from build123d import *

# Parameters (mm, degrees)
SKETCH1_W                            = 76.2
SKETCH1_H                            = 63.5
BOSS_EXTRUDE1_DEPTH                  = 14.2875
SKETCH2_W                            = 50.8
SKETCH2_H                            = 36.1
CUT_EXTRUDE1_DEPTH                   = 15.875
CUT_EXTRUDE2_DEPTH                   = 3.175
FILLET1_R                            = 3.175
F_4_40_TAPPED_HOLE1_D                = 2.2606
F_4_40_TAPPED_HOLE1_DEPTH            = 3.320847242
F_4_40_TAPPED_HOLE1_TIP              = 0.679152758
F_1_4_NPT_TAPPED_HOLE1_AT_2_COUNT    = 2
F_1_4_NPT_TAPPED_HOLE1_AT_2_PITCH    = 53.729845058
M10X1_5_TAPPED_HOLE1_D               = 8.5
M10X1_5_TAPPED_HOLE1_DEPTH           = 22.446342369
M10X1_5_TAPPED_HOLE1_TIP             = 2.553657631
M10X1_5_TAPPED_HOLE1_ON_FACE_2_D     = 8.5
M10X1_5_TAPPED_HOLE1_ON_FACE_2_DEPTH = 22.446342369
M10X1_5_TAPPED_HOLE1_ON_FACE_2_TIP   = 2.553657631
SKETCH16_W                           = 3.724215622
SKETCH16_H                           = 1.92405
FILLET2_R                            = 3.175
F_4_40_TAPPED_HOLE2_D                = 2.2606
F_4_40_TAPPED_HOLE2_DEPTH            = 6.920847242
F_4_40_TAPPED_HOLE2_TIP              = 0.679152758


with BuildPart() as part:
    # Sketch1 → Boss-Extrude1 (new body, symmetric)
    with BuildSketch(Plane(origin=(0, 0, 0), x_dir=(1, 0, 0), z_dir=(0, 1, 0))):
        Rectangle(SKETCH1_W, SKETCH1_H)
    extrude(amount=BOSS_EXTRUDE1_DEPTH, both=True)

    # Sketch2 → Cut-Extrude1 (cut)
    with BuildSketch(Plane(origin=(0, 14.2875, 0), x_dir=(1, 0, 0), z_dir=(0, 1, 0))):
        Rectangle(SKETCH2_W, SKETCH2_H)
    extrude(amount=-CUT_EXTRUDE1_DEPTH, mode=Mode.SUBTRACT)

    # Sketch3 → Cut-Extrude2 (cut)
    with BuildSketch(Plane(origin=(0, -1.5875, 0), x_dir=(1, 0, 0), z_dir=(0, 1, 0))):
        Polygon((-25.4, -7.05), (-14.4, -7.05), (-14.4, -18.05), (25.4, -18.05), (25.4, 7.05), (14.4, 7.05), (14.4, 18.05), (-25.4, 18.05), align=None)
    extrude(amount=-CUT_EXTRUDE2_DEPTH, mode=Mode.SUBTRACT)

    # Fillet1
    fillet1_edges = [part.edges().sort_by_distance(p)[0] for p in [
        (25.4, 6.35, -18.05),
        (25.4, 4.7625, 18.05),
        (-25.4, 6.35, 18.05),
        (-25.4, 4.7625, -18.05),
        (-14.4, -3.175, 18.05),
        (-14.4, -3.175, 7.05),
        (-25.4, -3.175, 7.05),
        (14.4, -3.175, -18.05),
        (14.4, -3.175, -7.05),
        (25.4, -3.175, -7.05),
    ]]
    fillet(fillet1_edges, radius=FILLET1_R)

    # #4-40 Tapped Hole1
    with Locations(Plane(origin=(10.9465, -4.7625, -11.6905), x_dir=(0, 0, 1), z_dir=(0, 1, 0))):
        with Locations((0, 0), (26.16, -7.493), (-2.779, -14.4), (23.381, -21.893)):
            Hole(F_4_40_TAPPED_HOLE1_D / 2, depth=F_4_40_TAPPED_HOLE1_DEPTH)
            with Locations((0, 0, -(F_4_40_TAPPED_HOLE1_DEPTH + F_4_40_TAPPED_HOLE1_TIP / 2))):  # 118° drill point
                Cone(0, F_4_40_TAPPED_HOLE1_D / 2, F_4_40_TAPPED_HOLE1_TIP, mode=Mode.SUBTRACT)

    # Sketch9 → 1/4 NPT Tapped Hole1 (revolve, cut)
    with BuildSketch(Plane(origin=(-22.225, -14.2875, 14.875), x_dir=(0, 0, -1), z_dir=(1, 0, 0))):
        Polygon((0, 0), (0, 26), (5.5626, 22.657652721), (5.5626, 10.02), (5.943676082, 10.02), (6.2436883, 0), align=None)
    f_1_4_npt_tapped_hole1 = revolve(axis=Axis((-22.225, -20.6375, 14.875), (0, 1, 0)), mode=Mode.SUBTRACT)

    # 1/4 NPT Tapped Hole1 at 2: 1/4 NPT Tapped Hole1 ×2
    with Locations(*[Vector(0.830543992, 0, -0.55695303) * (i * F_1_4_NPT_TAPPED_HOLE1_AT_2_PITCH) for i in range(1, F_1_4_NPT_TAPPED_HOLE1_AT_2_COUNT)]):
        add(f_1_4_npt_tapped_hole1, mode=Mode.SUBTRACT)

    # M10x1.5 Tapped Hole1
    with Locations(Plane(origin=(-21.9, 4.7625, -31.75), x_dir=(-1, 0, 0), z_dir=(0, 0, -1))):
        with Locations((0, 0)):
            Hole(M10X1_5_TAPPED_HOLE1_D / 2, depth=M10X1_5_TAPPED_HOLE1_DEPTH)
            with Locations((0, 0, -(M10X1_5_TAPPED_HOLE1_DEPTH + M10X1_5_TAPPED_HOLE1_TIP / 2))):  # 118° drill point
                Cone(0, M10X1_5_TAPPED_HOLE1_D / 2, M10X1_5_TAPPED_HOLE1_TIP, mode=Mode.SUBTRACT)

    # M10x1.5 Tapped Hole1 on face 2
    with Locations(Plane(origin=(21.9, 4.7625, 31.75), x_dir=(1, 0, 0), z_dir=(0, 0, 1))):
        with Locations((0, 0)):
            Hole(M10X1_5_TAPPED_HOLE1_ON_FACE_2_D / 2, depth=M10X1_5_TAPPED_HOLE1_ON_FACE_2_DEPTH)
            with Locations((0, 0, -(M10X1_5_TAPPED_HOLE1_ON_FACE_2_DEPTH + M10X1_5_TAPPED_HOLE1_ON_FACE_2_TIP / 2))):  # 118° drill point
                Cone(0, M10X1_5_TAPPED_HOLE1_ON_FACE_2_D / 2, M10X1_5_TAPPED_HOLE1_ON_FACE_2_TIP, mode=Mode.SUBTRACT)

    # Cut-Sweep1: sweep along a path in Sketch14
    with BuildLine(Plane(origin=(0, 14.2875, 0), x_dir=(1, 0, 0), z_dir=(0, 1, 0))) as cut_sweep1_path:
        Line((-21.4, 20.05), (21.4, 20.05))
        ThreePointArc((21.4, 20.05), (25.642640687, 18.292640687), (27.4, 14.05))
        Line((27.4, 14.05), (27.4, -14.05))
        ThreePointArc((27.4, -14.05), (25.642640687, -18.292640687), (21.4, -20.05))
        Line((21.4, -20.05), (-21.4, -20.05))
        ThreePointArc((-21.4, -20.05), (-25.642640687, -18.292640687), (-27.4, -14.05))
        Line((-27.4, -14.05), (-27.4, 14.05))
        ThreePointArc((-27.4, 14.05), (-25.642640687, 18.292640687), (-21.4, 20.05))
    # Sketch16 → Cut-Sweep1 (sweep, cut)
    with BuildSketch(Plane.XY):
        with Locations((-29.262107811, 13.325475)):
            Rectangle(SKETCH16_W, SKETCH16_H)
    sweep(path=cut_sweep1_path.line, mode=Mode.SUBTRACT)

    # Fillet2
    fillet2_edges = [part.edges().sort_by_distance(p)[0] for p in [
        (38.1, 0, 31.75),
        (-38.1, 0, 31.75),
        (-38.1, 0, -31.75),
        (38.1, 0, -31.75),
    ]]
    fillet(fillet2_edges, radius=FILLET2_R)

    # #4-40 Tapped Hole2
    with Locations(Plane(origin=(0, 14.2875, 0), x_dir=(1, 0, 0), z_dir=(0, 1, 0))):
        with Locations((34.124215622, 0), (30.228658441, 23.222452534), (-30.397379151, 23.047379151), (30.397379151, -23.047379151), (-30.397379151, -23.047379151), (0, -26.774215622), (-34.124215622, 0), (0.004913792, 26.774215622)):
            Hole(F_4_40_TAPPED_HOLE2_D / 2, depth=F_4_40_TAPPED_HOLE2_DEPTH)
            with Locations((0, 0, -(F_4_40_TAPPED_HOLE2_DEPTH + F_4_40_TAPPED_HOLE2_TIP / 2))):  # 118° drill point
                Cone(0, F_4_40_TAPPED_HOLE2_D / 2, F_4_40_TAPPED_HOLE2_TIP, mode=Mode.SUBTRACT)


solid = part.part
For this review, take the finished solid that the model builds, in its own axes (mm). A direction names the side the tool comes from. Give positions to 0.01 mm unless a question says otherwise; leave off trailing zeros. Loops run counter-clockwise (first coordinate to the right, second up) from the corner with the lowest first, then second, coordinate; pieces in that order, holes last. Notation, with made-up numbers: M 27,42 L 74,42 A7 cw 74,47 Z; hole C -3.75,17 d5. An arc over 180 degrees is marked long. Answer as a JSON object with one key per item and string values. Group by question number.
Q1. Add section B-B on z = 3. Give the boundary of the cut face in (x, y).
Q2. For probe 1 along Z at (x, y) = (5, 12); probe 2 along Z at (x, y) = (-21, 12.75); probe 3 along X at (y, z) = (-2, 0.5), list the stretches that pass through material, from the lowest coordinate up. Write a range as [from, to].
Q3. Add section A-A on y = -0.5. Give the boundary of the cut face in (x, z) (3 decimals), and give its area (3 significant figures).
Q4. Insertion check: P1, Ø7.5, axis at x = 21.9, y = 4.76, coming from the +Z side; P2, Ø15.5, axis at x = 15, z = -8.5, coming from the +Y side; P3, Ø5, axis at x = -21.9, y = 4.76, coming from the -Z side. Each pin has a flat end and moves straight along its axis. Give the tip position at first contact, or say it passes through.
Q5. Mouldability with a two-part tool opening along Z and no side actions: class faces 1 (the conical face through (24.641, 9.854, -17.181)), 2 (the flat face through (-38.1, 0, 0)) as +Z half, -Z half, draft (parallel to the pull), parting line (faces both ways), or undercut.
Q6. Tool access review of faces 3 (the cylindrical face through (0.147, 10.779, 25.654)), 4 (the flat face through (-1, -14.288, 0)): name each direction out of +Z, -Z, +X, -X, +Y, -Y from which nothing blocks a thin tool from reaching the whole face with its end or side.
Checked values:
{
 "1": {"outline": "M -38.1,-14.29 L 38.1,-14.29 L 38.1,14.29 L 31.12,14.29 L 31.12,12.36 L 27.4,12.36 L 27.4,14.29 L 25.4,14.29 L 25.4,-4.76 L -25.4,-4.76 L -25.4,14.29 L -27.4,14.29 L -27.4,12.36 L -31.12,12.36 L -31.12,14.29 L -38.1,14.29 Z"},
 "2": {"probe 1": "[-31.75, -18.05], [18.05, 31.75]", "probe 2": "[-31.75, -23.77], [-20.05, -18.05], [18.05, 20.05], [23.77, 31.75]", "probe 3": "[-38.1, -25.4], [25.4, 38.1]"},
 "3": {"outline": "M -38.1,-28.575 A3.175 ccw -34.925,-31.75 L 34.925,-31.75 A3.175 ccw 38.1,-28.575 L 38.1,28.575 A3.175 ccw 34.925,31.75 L -34.925,31.75 A3.175 ccw -38.1,28.575 Z; hole M -25.4,-14.875 A3.175 ccw -22.225,-18.05 L 17.716,-18.05 A5.563 ccw long 25.4,-10.366 L 25.4,14.875 A3.175 ccw 22.225,18.05 L -17.658,18.05 A5.563 ccw long -25.4,10.308 Z", "area": "2,940 mm²"},
 "4": {"P1": "z = 9", "P2": "y = -1.59", "P3": "z = 19.67"},
 "5": {"face 1": "undercut", "face 2": "draft"},
 "6": {"face 3": "+Y", "face 4": "+Z, -Z, +X, -X, -Y"}
}
